For this review, use the dimensioned drawing (mm, ordinates from the lowest corner) and the shaded views. A direction names the side the tool comes from. Round coordinates to 2 decimals unless told otherwise and drop trailing zeros. Order: outer loops, then holes, each group sorted by start corner. A loop starts at its lowest first (then second) coordinate and runs counter-clockwise, first axis right, second up. Notation, with made-up numbers: (66, -32) - (84, -32) arc R18 cw to (84, -1) - close; hole circle Ø2 at (80, -31.75). An arc over 180 degrees is marked (long way). Write item = value, one per line.
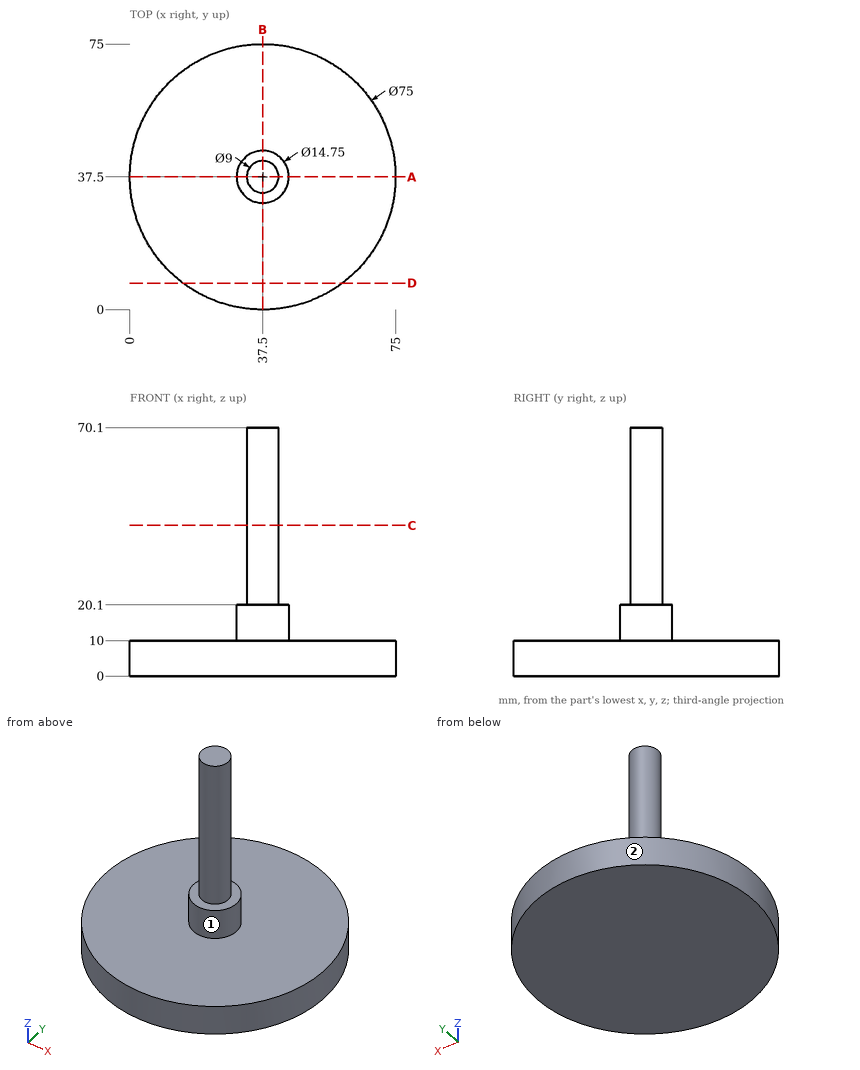
Item 1: Take a section at D-D, the plane y = 7.5. State the section outline as (x, z) points, and give its area (3 significant figures).
Data:
outline = (15, 0) - (60, 0) - (60, 10) - (15, 10) - close
area = 450 mm2
Item 2: Insertion check: P1, Ø3, axis at x = 23, y = 33, coming from the +Z side. The pin has a flat end and moves straight along its axis. Give the tip position at first contact, or say it passes through.
Data:
P1 = 10
Item 3: Take a section at A-A, the plane y = 37.5. State the section outline as (x, z) points (3 decimals).
Data:
outline = (0, 0) - (75, 0) - (75, 10) - (44.875, 10) - (44.875, 20.1) - (42, 20.1) - (42, 70.1) - (33, 70.1) - (33, 20.1) - (30.125, 20.1) - (30.125, 10) - (0, 10) - close
Item 4: Take a section at C-C, the plane z = 42.5. State the section outline as (x, y) points.
Data:
outline = circle Ø9 at (37.5, 37.5)
Item 5: For the marked faces 1 and 2, list the 3-axis set-ups (+Z, -Z, +X, -X, +Y, -Y) from which the entire face can be reached by the end or side of a thin tool; tool diameter is ignored.
Data:
face_1 = +Z
face_2 = +Z, -Z
Item 6: For line 1 along Z through (x, y) = (21.5, 18); line 2 along Z through (x, y) = (31.5, 38.5); line 3 along Y through (x, z) = (22, 5), list the stretches that pass through material, from the lowest coordinate up. Write a range as [from, to].
Data:
line_1 = [0, 10]
line_2 = [0, 20.1]
line_3 = [3.35, 71.65]
